Here's how the part is built. I have some questions about the finished solid (model axes, mm). Coordinates: 2 decimals unless noted, no trailing zeros. Write each loop counter-clockwise with the first axis right and the second up, starting at its lowest first coordinate (ties: lowest second). Pieces come first, ordered by that corner, then holes.
(1) Imagine slicing it at C-C, the plane z = 0.15. State how many separate pieces and enclosed holes the cut face has, plus the area to 3 significant figures.
(2) Imagine slicing it at B-B, the plane x = 40. List the corners of the cut face in (y, z) for me, plus the area to 3 significant figures.
(3) Please list where these lines run through material, in increasing order: probe 1 along X at (y, z) = (-13.5, -0.95); probe 2 along Y at (x, z) = (48, -0.85); probe 3 along Y at (x, z) = (-52.5, -2.05).
(4) For pin 1 Ø2.5 at (y, z) = (0, 1) entering from +X; pin 2 Ø3.5 at (x, y) = (-48.79, 51.45) entering from +Z; pin 3 Ø1.5 at (y, z) = (45, 1) entering from +X; pin 4 Ø1 at (x, z) = (35.5, 1) entering from -Y, each with a flat end and sliding along its axis, tell me the tip position at first contact or that it passes through.
(5) Imagine slicing it at A-A, the plane x = 0. List the corners of the cut face in (y, z) for me.
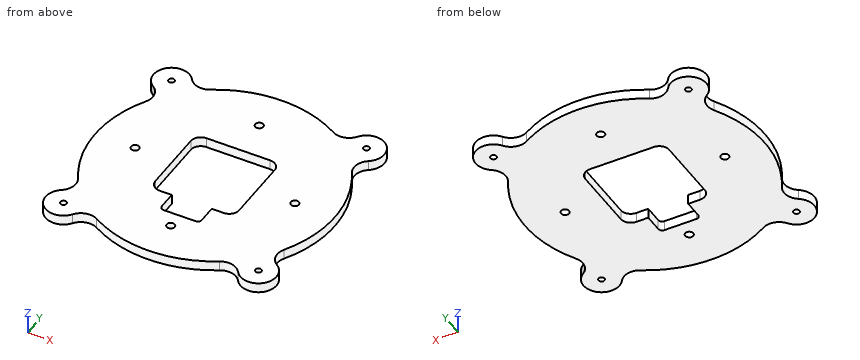
```python
from build123d import *

# Parameters (mm, degrees)
SKETCH1_R             = 1.5
SKETCH1_R_2           = 2
BOSS_EXTRUDE1_DEPTH   = 5
BODY_MOVE_COPY1_ANGLE = 90


with BuildPart() as part:
    # Sketch1 → Boss-Extrude1 (new body)
    with BuildSketch(Plane(origin=(0, 0, 0), x_dir=(1, 0, 0), z_dir=(0, 1, 0))):
        with BuildLine():
            ThreePointArc((41.376602734, 53.892924716), (36.497232574, 50.613564399), (30.69404934, 51.554585976))
            ThreePointArc((30.69404934, 51.554585976), (0, 60), (-30.69404934, 51.554585976))
            ThreePointArc((-30.69404934, 51.554585976), (-36.497232574, 50.613564399), (-41.376602734, 53.892924716))
            ThreePointArc((-41.376602734, 53.892924716), (-55.154328933, 55.154328933), (-53.892924716, 41.376602734))
            ThreePointArc((-53.892924716, 41.376602734), (-50.613564399, 36.497232574), (-51.554585976, 30.69404934))
            ThreePointArc((-51.554585976, 30.69404934), (-60, 0), (-51.554585976, -30.69404934))
            ThreePointArc((-51.554585976, -30.69404934), (-50.613564399, -36.497232574), (-53.892924716, -41.376602734))
            ThreePointArc((-53.892924716, -41.376602734), (-55.154328933, -55.154328933), (-41.376602734, -53.892924716))
            ThreePointArc((-41.376602734, -53.892924716), (-36.497232574, -50.613564399), (-30.69404934, -51.554585976))
            ThreePointArc((-30.69404934, -51.554585976), (0, -60), (30.69404934, -51.554585976))
            ThreePointArc((30.69404934, -51.554585976), (36.497232574, -50.613564399), (41.376602734, -53.892924716))
            ThreePointArc((41.376602734, -53.892924716), (55.154328933, -55.154328933), (53.892924716, -41.376602734))
            ThreePointArc((53.892924716, -41.376602734), (50.613564399, -36.497232574), (51.554585976, -30.69404934))
            ThreePointArc((51.554585976, -30.69404934), (60, 0), (51.554585976, 30.69404934))
            ThreePointArc((51.554585976, 30.69404934), (50.613564399, 36.497232574), (53.892924716, 41.376602734))
            ThreePointArc((53.892924716, 41.376602734), (55.154328933, 55.154328933), (41.376602734, 53.892924716))
        make_face()
        with Locations((-48.790367902, -48.790367902)):
            Circle(SKETCH1_R, mode=Mode.SUBTRACT)
        with Locations((0, -40)):
            Circle(SKETCH1_R_2, mode=Mode.SUBTRACT)
        with Locations((48.790367902, -48.790367902)):
            Circle(SKETCH1_R, mode=Mode.SUBTRACT)
        with BuildLine():
            Line((16.001917019, -21), (10, -21))
            Line((10, -21), (10, -30.000108076))
            ThreePointArc((10, -30.000108076), (9.414180319, -31.414301502), (7.999957489, -32.000050194))
            Line((7.999957489, -32.000050194), (-8.000158272, -32.000050194))
            ThreePointArc((-8.000158272, -32.000050194), (-9.414280711, -31.414259919), (-10, -30.000108076))
            Line((-10, -30.000108076), (-10, -21))
            Line((-10, -21), (-16.005742178, -21))
            ThreePointArc((-16.005742178, -21), (-19.538404995, -19.534344662), (-21, -16))
            Line((-21, -16), (-21, 16))
            ThreePointArc((-21, 16), (-19.535533906, 19.535533906), (-16, 21))
            Line((-16, 21), (16, 21))
            ThreePointArc((16, 21), (19.535388079, 19.536388365), (21.000355251, 16.001561768))
            Line((21.000355251, 16.001561768), (21.000355251, -16.001561768))
            ThreePointArc((21.000355251, -16.001561768), (19.536346588, -19.535991337), (16.001917019, -21))
        make_face(mode=Mode.SUBTRACT)
        with Locations((40, 0)):
            Circle(SKETCH1_R_2, mode=Mode.SUBTRACT)
        with Locations((-40, 0)):
            Circle(SKETCH1_R_2, mode=Mode.SUBTRACT)
        with Locations((-48.790367902, 48.790367902)):
            Circle(SKETCH1_R, mode=Mode.SUBTRACT)
        with Locations((0, 40)):
            Circle(SKETCH1_R_2, mode=Mode.SUBTRACT)
        with Locations((48.790367902, 48.790367902)):
            Circle(SKETCH1_R, mode=Mode.SUBTRACT)
    extrude(amount=BOSS_EXTRUDE1_DEPTH)


with BuildPart() as part_1:
    # Body-Move/Copy1: moved
    add(part.part.rotate(Axis((0, 2.5, 0.160861545), (1, 0, 0)), BODY_MOVE_COPY1_ANGLE))


solid = part_1.part
```
Recorded:
1. separate pieces: 1
1. enclosed holes: 9
1. area: 10,500 mm2
2. outline: (-49.7, -2.34) - (0.66, -2.34) - (0.66, 2.66) - (-49.7, 2.66) - close; (4.66, -2.34) - (55.02, -2.34) - (55.02, 2.66) - (4.66, 2.66) - close
2. area: 504 mm2
3. probe 1: x = -57.78 to -21, 21 to 57.78
3. probe 2: y = -55.09 to -47.4, -44.85 to 50.18, 52.73 to 60.42
3. probe 3: y = -54.33 to -37.5, -26.39 to 31.71, 42.82 to 59.65
4. pin 1: stops at x = 59.98
4. pin 2: stops at z = 2.66
4. pin 3: stops at x = 55.75
4. pin 4: stops at y = -47.86
5. outline: (-57.34, -2.34) - (-39.34, -2.34) - (-39.34, 2.66) - (-57.34, 2.66) - close; (-35.34, -2.34) - (-29.34, -2.34) - (-29.34, 2.66) - (-35.34, 2.66) - close; (23.66, -2.34) - (40.66, -2.34) - (40.66, 2.66) - (23.66, 2.66) - close; (44.66, -2.34) - (62.66, -2.34) - (62.66, 2.66) - (44.66, 2.66) - close
